Model file for the job. Use its own axes, mm. Give positions to 0.01 mm unless a question says otherwise; leave off trailing zeros. Order: outer loops, then holes, each group sorted by start corner. A loop starts at its lowest first (then second) coordinate and runs counter-clockwise, first axis right, second up. Notation, with made-up numbers: (-10.5, -6.5) - (43.5, -6.5) arc R21 cw to (43.5, -0.5) - close; hole circle Ø11 at (21, 26.5). An arc over 180 degrees is marked (long way). Use CSV: the item, a comma, the result in double quotes. Start each with the question number.
(1) Probe L1, parallel to X at y = 71, z = 11; L2, parallel to X at y = 54.5, z = 17; L3, parallel to Y at x = 37, z = 7. List the from-to ranges inside material, lowest first.
(2) Band-saw the part on A-A, the plane z = 33. Give the cut face in (x, y), then the cut area to 3 significant figures.
(3) Band-saw the part on C-C, the plane x = 59. Give the cut face in (y, z), then the cut area to 3 significant figures.
(4) Drop flat-ended pins along their axis: pin 1 Ø1 at (x, z) = (67, 24.5) entering from -Y; pin 2 Ø4 at (x, y) = (35, 69.5) entering from -Z; pin 3 Ø12 at (y, z) = (52.5, 9) entering from -X; pin 4 Ø10 at (y, z) = (68, 10.5) entering from +X. Give the stop position or say it passes through.
(5) Band-saw the part on B-B, the plane z = 17. Give the cut face in (x, y).
(6) Band-saw the part on D-D, the plane y = 57. Give the cut face in (x, z).
from build123d import *

# Parameters (mm, degrees)
ESTRUSIONE_ESTRUSIONE1_DEPTH      = 46
ESTRUSIONE_ESTRUSIONE1_DEPTH_BACK = 2
SCHIZZO2_W                        = 10
SCHIZZO2_H                        = 46
SCHIZZO2_W_2                      = 18
ESTRUSIONE_ESTRUSIONE2_DEPTH      = 2
SCHIZZO3_W                        = 40
SCHIZZO3_H                        = 27
TAGLIO_ESTRUSIONE1_DEPTH          = 10
RACCORDO1_R                       = 4


with BuildPart() as part:
    # Schizzo1 → Estrusione-Estrusione1 (new, two sides: drawn at the far end of the back side and taken through both)
    with BuildSketch(Plane.XY.offset(-ESTRUSIONE_ESTRUSIONE1_DEPTH_BACK)):
        Polygon((62.384284835, 50.597287007), (38.536156503, 68.79802257), (37.322774132, 67.208147347), (61.170902464, 49.007411784), align=None)
    extrude(amount=ESTRUSIONE_ESTRUSIONE1_DEPTH + ESTRUSIONE_ESTRUSIONE1_DEPTH_BACK)

    # Schizzo2 → Estrusione-Estrusione2 (add)
    with BuildSketch(Plane(origin=(46.150805657, 60.470651428, 0), x_dir=(0.7949376110826004, -0.606691185436453, 0), z_dir=(-0.606691185436453, -0.7949376110826004, 0))):
        with Locations((-16.105313678, 23)):
            Rectangle(SCHIZZO2_W, SCHIZZO2_H)
        with Locations((27.894686322, 23)):
            Rectangle(SCHIZZO2_W_2, SCHIZZO2_H)
    extrude(amount=-ESTRUSIONE_ESTRUSIONE2_DEPTH)

    # Schizzo3 → Taglio-Estrusione1 (cut)
    with BuildSketch(Plane(origin=(47.364188028, 62.06052665, 0), x_dir=(0.7949376110826014, -0.6066911854364516, 0), z_dir=(0.6066911854364516, 0.7949376110826014, 0))):
        with Locations((7.894686322, -32.5)):
            Rectangle(SCHIZZO3_W, SCHIZZO3_H)
    extrude(amount=-TAGLIO_ESTRUSIONE1_DEPTH, mode=Mode.SUBTRACT)

    # Raccordo1
    raccordo1_edges = [part.edges().sort_by_distance(p)[0] for p in [
        (37.134527706, 68.609776144, 19),
        (68.932032149, 44.342128727, 19),
    ]]
    fillet(raccordo1_edges, radius=RACCORDO1_R)


solid = part.part
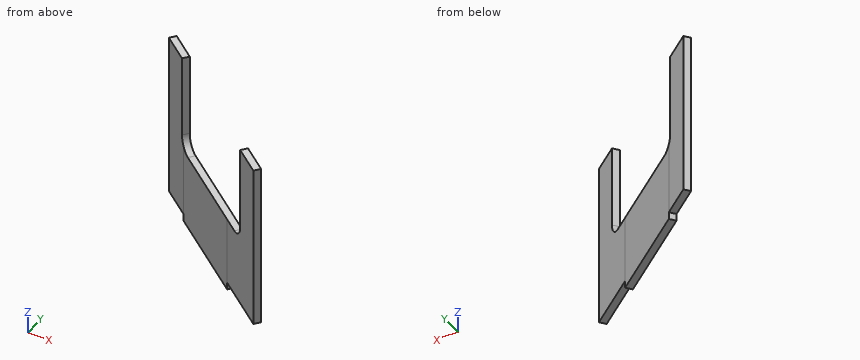
Answer block:
1,L1,"x = 32.35 to 35.65"
1,L2,"x = 53.97 to 57.27"
1,L3,"y = 67.45 to 69.97"
2,outline,"(29.37, 73.28) - (36.53, 67.81) - (37.74, 69.4) - (30.59, 74.86) - close; (68.33, 43.55) - (75.48, 38.09) - (76.69, 39.68) - (69.54, 45.14) - close"
2,area,"36.0 mm2"
3,outline,"(50.66, -2) - (53.18, -2) - (53.18, 19) - (50.66, 19) - close"
3,area,"52.8 mm2"
4,pin 1,"passes through"
4,pin 2,"stops at z = 0"
4,pin 3,"stops at x = 48.73"
4,pin 4,"stops at x = 46.13"
5,outline,"(29.37, 73.28) - (75.48, 38.09) - (76.69, 39.68) - (30.59, 74.86) - close"
6,outline,"(50.7, -2) - (53.99, -2) - (53.99, 19) - (50.7, 19) - close"
